CAD build for the part. Positions are in the model's coordinates, mm. A direction names the side the tool comes from. Round coordinates to 2 decimals unless told otherwise and drop trailing zeros. Loops run counter-clockwise (first coordinate to the right, second up) from the corner with the lowest first, then second, coordinate; pieces in that order, holes last. Notation, with made-up numbers: (86.25, 49) - (112.25, 49) arc R14 cw to (112.25, 71) - close; hole circle Ø10 at (47, 29). An arc over 180 degrees is marked (long way). One line per question, with ' | ' between items.
Autodesk Inventor part; units mm, degrees
ref_plane "YZ Plane" through (0, 0, 0) normal (1, 0, 0) x (0, 1, 0)
ref_plane "XZ Plane" through (0, 0, 0) normal (0, 1, 0) x (-1, 0, 0)
ref_plane "XY Plane" through (0, 0, 0) normal (0, 0, 1) x (1, 0, 0)
sketch "Sketch1" plane through (0, 0, 0) normal (0, 1, 0) x (-1, 0, 0)
  circle A0 centre (0, 0) radius 5
  circle A1 centre (0, 0) radius 9
  dimension "d0" = 10
  dimension "d1" = 4
extrude "Extrusion1" add sketch "Sketch1" along normal blind 28
sketch "Sketch2" plane through (0, 0, 0) normal (0, 0, 1) x (1, 0, 0)
  line L0 (9, 28) -> (-9, 28)
  line L1 (0, 28) -> (0, 0)
  circle A0 centre (0, 14) radius 1.8
  dimension "d4" = 3.6
extrude "Extrusion2" cut sketch "Sketch2" along normal mid plane 20
sketch "Sketch4" plane through (0, 28, 0) normal (0, 1, 0) x (1, 0, 0)
  line L0 (2.1794, 4.5) -> (-2.1794, 4.5)
  arc A0 (2.1794, 4.5) -> (-2.1794, 4.5) centre (0, 0) ccw
extrude "Extrusion3" add sketch "Sketch4" against normal blind 11
properties part number "shaft_connector"
(1) Drop flat-ended pins along their axis: P1, Ø4, axis at y = 11.5, z = -6, coming from the -X side; P2, Ø1, axis at x = 1, y = 18, coming from the +Z side; P3, Ø2, axis at x = 0, y = 14, coming from the -Z side; P4, Ø3, axis at y = 16, z = -4, coming from the -X side. Give the stop position or say it passes through.
Results found:
P1: stops at x = -8.06 | P2: stops at z = 8.99 | P3: passes through | P4: stops at x = -8.65
(2) Cut at D-D, the plane y = 10.25. Write the cut outline in (x, z), then the cut area to 3 significant figures.
Results found:
outline: circle Ø18 at (0, 0); hole circle Ø10 at (0, 0) | area: 176 mm²
(3) Probe L1, parallel to Y at x = 0, z = -7.95; L2, parallel to Z at x = 0, y = 4.5; L3, parallel to X at y = 17.75, z = -2.75. List the from-to ranges inside material, lowest first.
Results found:
L1: y = 0 to 12.2, 15.8 to 28 | L2: z = -9 to -5, 5 to 9 | L3: x = -8.57 to -4.18, 4.18 to 8.57
(4) Cut at B-B, the plane z = 0. Write the cut outline in (x, y), then the cut area to 3 significant figures.
Results found:
outline: (-9, 0) - (-5, 0) - (-5, 28) - (-9, 28) - close; (5, 0) - (9, 0) - (9, 28) - (5, 28) - close | area: 224 mm²
(5) Tool access for faces 4 (the face through (0, 23, -4.5)), 5 (the face through (1.717, 14.541, 6.863)): list every direction of +Z, -Z, +X, -X, +Y, -Y with a clear straight run to the whole face (end or side of a thin tool).
Results found:
face 4: +Y, -Y | face 5: +Z, -Z
(6) Cut at C-C, the plane x = 3. Write the cut outline in (y, z).
Results found:
outline: (0, -8.49) - (28, -8.49) - (28, -4) - (0, -4) - close; (0, 4) - (28, 4) - (28, 8.49) - (0, 8.49) - close
(7) Two-plate mould, pull along Y, no slides. Class faces 1 (the face through (-1.8, 14.08, -6.8)), 2 (the face through (1.951, 13.804, 8.786)), 3 (the face through (-4, 0, -4)): released by +Y, released by -Y, zero draft, split by the parting line, or undercut.
Results found:
face 1: undercut | face 2: zero draft | face 3: released by -Y
(8) Cut at A-A, the plane x = 0. Write the cut outline in (y, z), then the cut area to 3 significant figures.
Results found:
outline: (0, -9) - (12.2, -9) - (12.2, -5) - (0, -5) - close; (0, 5) - (12.2, 5) - (12.2, 9) - (0, 9) - close; (15.8, -9) - (28, -9) - (28, -4.5) - (17, -4.5) - (17, -5) - (15.8, -5) - close; (15.8, 5) - (28, 5) - (28, 9) - (15.8, 9) - close | area: 201 mm²
